Verification items for the finished model (mm, model axes). A direction names the side the tool comes from. Coordinates: 2 decimals unless noted, no trailing zeros. Write each loop counter-clockwise with the first axis right and the second up, starting at its lowest first coordinate (ties: lowest second). Pieces come first, ordered by that corner, then holes. Notation, with made-up numbers: M -3,47.5 L 30,47.5 A24 ccw 30,69.5 Z; hole C -40,8 d6. An arc over 180 degrees is marked long. One line per item, written item: value.
```python
from build123d import *

# Parameters (mm, degrees)
BOSS_EXTRUDE1_DEPTH = 10
BOSS_EXTRUDE1_DRAFT = 8


with BuildPart() as part:
    # Sketch1 → Boss-Extrude1 (with draft: the straight prism first)
    with BuildSketch(Plane(origin=(0, 0, 0), x_dir=(1, 0, 0), z_dir=(0, 1, 0))):
        with BuildLine():
            Line((36.892843318, -6.916769299), (25.392844844, -6.907371064))
            ThreePointArc((25.392844844, -6.907371064), (17.862146893, -24.595305322), (0.029881046, -31.777555993))
            ThreePointArc((0.029881046, -31.777555993), (-17.799721033, -24.588695191), (-25.323861346, -6.897970432))
            Line((-25.323861346, -6.897970432), (-36.823861346, -6.897970432))
            ThreePointArc((-36.823861346, -6.897970432), (0.025091553, -43.765722197), (36.892843318, -6.916769299))
        make_face()
    extrude(amount=BOSS_EXTRUDE1_DEPTH)
    # Boss-Extrude1: the draft: its side faces are tilted about the plane it starts from
    boss_extrude1_sides = [part.faces().sort_by_distance(p)[0] for p in [
        (31.142844081, 5, 6.912070181),
        (17.862146893, 5, 24.595305322),
        (-17.799721033, 5, 24.588695191),
        (-31.073861346, 5, 6.897970432),
        (0.025091553, 5, 43.765722197),
    ]]
    draft(boss_extrude1_sides, Plane(origin=(0, 0, 0), x_dir=(1, 0, 0), z_dir=(0, 1, 0)), BOSS_EXTRUDE1_DRAFT)

    # Chamfer3: read off the stored shape, not the designer's step
    # Chamfer3 outline → Chamfer3 (revolve, cut)
    with BuildSketch(Plane(origin=(-0.207197369, 0, 6.660892016), x_dir=(1, 0, 0), z_dir=(0, 0, 1))):
        Polygon((25.131460191, 10), (25.131460191, 0.097319313), (30.62060573, 10), align=None)
    revolve(axis=Axis((-0.207197369, 0, 6.660892016), (0, 1, 0)), mode=Mode.SUBTRACT)

    # Chamfer3 2 outline → Chamfer3 2 (revolve, cut)
    with BuildSketch(Plane(origin=(0.27627048, 0, 6.66098163), x_dir=(1, 0, 0), z_dir=(0, 0, 1))):
        Polygon((25.295653078, 1.265612408), (25.131460191, 0.097319313), (30.62060573, 10), (25.295653078, 10), align=None)
    revolve(axis=Axis((0.27627048, 0, 6.66098163), (0, 1, 0)), mode=Mode.SUBTRACT)


solid = part.part
```
Item 1: Access from +Z, -Z, +X, -X, +Y, -Y to the whole of each face (thin tool, end or side, straight path). Record for faces 4 (the face through (19.172, 4.018, 26.371)), 5 (the face through (0, 0, 33)).
The answers:
face 4: -Z, +Y
face 5: +Z, -Z, +X, -X, -Y
Item 2: Scan lines: line 1 (X direction, y = 1.5, z = 20); line 2 (X direction, y = 9.25, z = 17); line 3 (Z direction, x = 14, y = 8.5). Record each from-to range of solid material in increasing order.
The answers:
line 1: x = -34.19 to -22.42, 22.49 to 34.26
line 2: x = -34.06 to -28.59, 28.66 to 34.13
line 3: z = 33.1 to 39.72
Item 3: Go/stop test with flat-tipped pins: P1, Ø10, axis at x = -18, z = 20, coming from the -Y side; P2, Ø5, axis at y = 5, z = 14.5, coming from the +X side; P3, Ø4, axis at y = 6, z = 19.5, coming from the +X side; P4, Ø5, axis at x = 22, y = 2.5, coming from the +Z side. Record where each tip stops, or that it passes through.
The answers:
P1: stops at y = 0
P2: stops at x = 35.97
P3: stops at x = 34.52
P4: stops at z = 37.85
Item 4: Draft check along X on faces 1 (the face through (-32.271, 3.819, 7.435)), 2 (the face through (-19.539, 4.018, 25.943)), 3 (the face through (-0.763, 7.152, 42.752)). Enter one of: released by +X, released by -X, zero draft, split by the parting line, or undercut.
The answers:
face 1: zero draft
face 2: undercut
face 3: split by the parting line
Item 5: Cross-section at B-B, the plane y = 9.25. Enter the section's corners in (x, z), and give its area (3 significant figures).
The answers:
outline: M -35.5,8.2 L -30.37,8.2 A30.2 cw 0.03,36.86 A30.2 cw 30.44,8.21 L 35.57,8.22 A35.56 ccw Z
area: 540 mm²
